Could you check a few things on this model? Use its own coordinates, in mm. Face numbers are marked on the shaded views. Round coordinates to 2 decimals unless told otherwise and drop trailing zeros. Write each loop counter-clockwise with the first axis right and the second up, starting at its lowest first coordinate (ties: lowest second). Pieces come first, ordered by that corner, then holes. Notation, with made-up numbers: M -2,46.5 L 13,46.5 A21 ccw 13,84.5 Z; hole C -31,57 d4. An arc over 180 degrees is marked long. One line per item, written item: value. Start each with the question number.
(1) I want a section at C-C on z = -50.8. Please give me the cut outline in (x, y), and give its area (3 significant figures).
(2) I want a section at B-B on x = 95.25. Please give me the cut outline in (y, z) (3 decimals).
(3) I want a section at D-D on x = 57. Please give me the cut outline in (y, z).
(4) I'm going to push a flat-ended pin straight in: pin 1 Ø6.5 at (x, z) = (74.37, -25.78) entering from -Y. Where does the tip first touch, or does it pass through?
(5) I want a section at A-A on z = -93.98. Please give me the cut outline in (x, y) (3 decimals), and give its area (3 significant figures).
(6) Thinking about a two-plate mould opening in X: for the marked faces 1, 2 and 3, which applies, released by +X, released by -X, zero draft, split by the parting line, or undercut?
(7) If I drill on L1, parallel to Z at x = 6, y = 5.25; L2, parallel to Z at x = 50.8, y = 6.25; L3, parallel to X at y = -0.5, z = -29.5, over which ranges is the centre line in solid material (lowest first)?
```python
from build123d import *

# Parameters (mm, degrees)
SKETCH1_W           = 101.6
SKETCH1_H           = 101.6
SKETCH1_R           = 2.54
SKETCH1_R_2         = 14.097
BOSS_EXTRUDE1_DEPTH = 7.62
SKETCH1_3_W         = 12.7
SKETCH1_3_H         = 101.6
BOSS_EXTRUDE2_DEPTH = 7.62
SKETCH3_R           = 3.175
CUT_EXTRUDE1_DEPTH  = 25.4


with BuildPart() as part:
    # Sketch1 → Boss-Extrude1 (new body)
    with BuildSketch(Plane(origin=(0, 0, 0), x_dir=(1, 0, 0), z_dir=(0, 1, 0))):
        with Locations((50.8, 50.8)):
            Rectangle(SKETCH1_W, SKETCH1_H)
        with Locations(Location((27.2288, 75.819, 0), (0, 0, 90))):
            Circle(SKETCH1_R, mode=Mode.SUBTRACT)
        with Locations(Location((74.3712, 75.819, 0), (0, 0, 90))):
            Circle(SKETCH1_R, mode=Mode.SUBTRACT)
        with Locations(Location((27.2288, 25.781, 0), (0, 0, 90))):
            Circle(SKETCH1_R, mode=Mode.SUBTRACT)
        with Locations(Location((74.3712, 25.781, 0), (0, 0, 90))):
            Circle(SKETCH1_R, mode=Mode.SUBTRACT)
        with Locations(Location((50.8, 50.8, 0), (0, 0, 90))):
            Circle(SKETCH1_R_2, mode=Mode.SUBTRACT)
    extrude(amount=BOSS_EXTRUDE1_DEPTH)

    # Sketch1_3 → Boss-Extrude2 (add)
    with BuildSketch(Plane(origin=(0, 0, 0), x_dir=(1, 0, 0), z_dir=(0, 1, 0))):
        Polygon((0, 101.6), (0, 0), (12.7, 12.7), (12.7, 101.6), align=None)
        Polygon((12.7, 12.7), (0, 0), (12.7, 0), align=None)
        with Locations((95.25, 50.8)):
            Rectangle(SKETCH1_3_W, SKETCH1_3_H)
    extrude(amount=-BOSS_EXTRUDE2_DEPTH)

    # Sketch3 → Cut-Extrude1 (cut)
    with BuildSketch(Plane.XZ.offset(7.62)):
        with Locations(Location((6.35, -7.62, 0), (0, 0, 270))):
            Circle(SKETCH3_R)
        with Locations(Location((95.25, -7.62, 0), (0, 0, 270))):
            Circle(SKETCH3_R)
        with Locations(Location((6.35, -93.98, 0), (0, 0, 270))):
            Circle(SKETCH3_R)
        with Locations(Location((95.25, -93.98, 0), (0, 0, 270))):
            Circle(SKETCH3_R)
    extrude(amount=-CUT_EXTRUDE1_DEPTH, mode=Mode.SUBTRACT)


solid = part.part
```
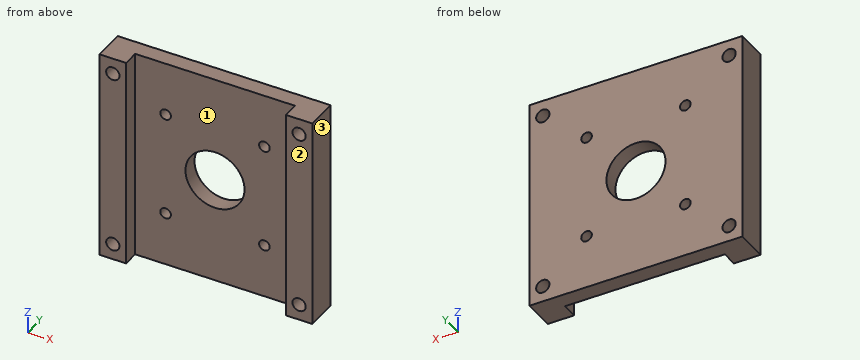
Found:
1. outline: M 0,-7.62 L 12.7,-7.62 L 12.7,0 L 36.7,0 L 36.7,7.62 L 0,7.62 Z; M 64.9,0 L 88.9,0 L 88.9,-7.62 L 101.6,-7.62 L 101.6,7.62 L 64.9,7.62 Z
1. area: 753 mm²
2. outline: M -7.62,-101.6 L 7.62,-101.6 L 7.62,-97.155 L -7.62,-97.155 Z; M -7.62,-90.805 L 7.62,-90.805 L 7.62,-10.795 L -7.62,-10.795 Z; M -7.62,-4.445 L 7.62,-4.445 L 7.62,0 L -7.62,0 Z
3. outline: M 0,-101.6 L 7.62,-101.6 L 7.62,-63.46 L 0,-63.46 Z; M 0,-38.14 L 7.62,-38.14 L 7.62,0 L 0,0 Z
4. pin 1: stops at y = 0
5. outline: M 0,-7.62 L 3.175,-7.62 L 3.175,7.62 L 0,7.62 Z; M 9.525,-7.62 L 12.7,-7.62 L 12.7,0 L 88.9,0 L 88.9,-7.62 L 92.075,-7.62 L 92.075,7.62 L 9.525,7.62 Z; M 98.425,-7.62 L 101.6,-7.62 L 101.6,7.62 L 98.425,7.62 Z
5. area: 774 mm²
6. face 1: undercut
6. face 2: zero draft
6. face 3: released by +X
7. L1: z = -101.6 to -97.14, -90.82 to -10.78, -4.46 to 0
7. L2: z = -101.6 to -64.9, -36.7 to 0
7. L3: x = 0 to 12.7, 88.9 to 101.6
